```python
from build123d import *

# Parameters (mm, degrees)
SKETCH_R           = 64
PAD_DEPTH          = 4
PAD001_DEPTH       = 50
POLARPATTERN_COUNT = 3
SKETCH002_R        = 64
PAD002_DEPTH       = 4


with BuildPart() as part:
    # Sketch → Pad (new body)
    with BuildSketch(Plane.XY):
        Circle(SKETCH_R)
    extrude(amount=-PAD_DEPTH)

    # Sketch001 → Pad001 (join)
    with BuildSketch(Plane.XY):
        with BuildLine():
            ThreePointArc((29, 19.052559), (29, -19.052559), (62, 0))
            ThreePointArc((62, 0), (60, 2), (58, 0))
            ThreePointArc((31, 15.588457), (31, -15.588457), (58, 0))
            ThreePointArc((31, 15.588457), (41.999973, 34.641035), (30.99994, 53.693578))
            ThreePointArc((30.99994, 53.693578), (28.267891, 52.961523), (28.999946, 50.229473))
            ThreePointArc((29, 19.052559), (37.999973, 34.641032), (28.999946, 50.229473))
        make_face()
    pad001 = extrude(amount=PAD001_DEPTH)

    # PolarPattern: Pad001 ×3 about axis
    polarpattern_axis = Axis((0, 0, 0), (0, 0, 1))
    for i in range(1, POLARPATTERN_COUNT):
        add(pad001.rotate(polarpattern_axis, i * 360 / POLARPATTERN_COUNT))

    # Sketch002 → Pad002 (join)
    with BuildSketch(Plane.XY.offset(50)):
        Circle(SKETCH002_R)
    extrude(amount=PAD002_DEPTH)


solid = part.part
```
The model under review builds one solid part; all positions refer to its coordinate system, in mm. A direction names the side the tool comes from. Round coordinates to 2 decimals unless told otherwise and drop trailing zeros. Order: outer loops, then holes, each group sorted by start corner. A loop starts at its lowest first (then second) coordinate and runs counter-clockwise, first axis right, second up.
(1) Take a section at D-D, the plane x = -12.5. State the section outline as (y, z) points, plus the area to 3 significant figures.
Working result:
outline: (-62.77, -4) - (62.77, -4) - (62.77, 0) - (55.32, 0) - (55.32, 50) - (62.77, 50) - (62.77, 54) - (-62.77, 54) - (-62.77, 50) - (-18.28, 50) - (-18.28, 0) - (-62.77, 0) - close; hole (-13.96, 0) - (13.96, 0) - (13.96, 50) - (-13.96, 50) - close; hole (18.28, 0) - (51, 0) - (51, 50) - (18.28, 50) - close
area: 1,650 mm2
(2) Take a section at A-A, the plane z = 46. State the section outline as (x, y) points.
Working result:
outline: (-62, 0) arc R2 ccw to (-58, 0) arc R18 cw to (-31, 15.59) arc R22 ccw (long way) to (-31, 53.69) arc R2 ccw to (-29, 50.23) arc R18 cw (long way) to (-29, 19.05) arc R22 ccw to start; (-31, -53.69) arc R2 ccw to (-29, -50.23) arc R18 cw (long way) to (-2, -34.64) arc R22 ccw to (31, -53.69) arc R2 ccw to (29, -50.23) arc R18 cw to (2, -34.64) arc R22 ccw (long way) to start; (29, 19.05) arc R22 ccw (long way) to (62, 0) arc R2 ccw to (58, 0) arc R18 cw (long way) to (31, 15.59) arc R22 ccw to (31, 53.69) arc R2 ccw to (29, 50.23) arc R18 cw to start
(3) For P1, Ø1, axis at x = -14, z = 21.5, coming from the -Y side; P2, Ø1.5, axis at y = 49.5, z = 28, coming from the +X side, all flat-tipped, find the tip position at first contact; note any pin that passes through.
Working result:
P1: stops at y = -17.86
P2: stops at x = 36.88
(4) Take a section at C-C, the plane y = 24. State the section outline as (x, z) points.
Working result:
outline: (-59.33, -4) - (59.33, -4) - (59.33, 0) - (39.26, 0) - (39.26, 50) - (59.33, 50) - (59.33, 54) - (-59.33, 54) - (-59.33, 50) - (-5.48, 50) - (-5.48, 0) - (-59.33, 0) - close; hole (-0.74, 0) - (34.52, 0) - (34.52, 50) - (-0.74, 50) - close
(5) Wall thickness on L1, parallel to Y at x = -20, z = 18; L2, parallel to Z at x = -47, y = 3; L3, parallel to X at y = -0.5, z = 22: over which ranges is each line inside the solid? List them lowest first.
Working result:
L1: y = -16.64 to -12.64, 12.64 to 16.64, 52.64 to 56.64
L2: z = -4 to 0, 50 to 54
L3: x = -61.94 to -58.06, 18.01 to 22.01, 57.99 to 61.99
(6) Mouldability with a two-part tool opening along Y and no side actions: class faces 1 (the face through (-60, -2, 25)), 2 (the face through (-13.87, -62.48, -1.97)), 3 (the face through (-1, 1, 50)), 4 (the face through (1.99, 34, 24.65)) as released by +Y, released by -Y, zero draft, split by the parting line, or undercut.
Working result:
face 1: released by -Y
face 2: split by the parting line
face 3: undercut
face 4: undercut
(7) Tool access review of faces 5 (the face through (41.998, 34.319, 24.65)), 6 (the face through (-2.008, 34.113, 24.65)), 7 (the face through (60, 2, 25)): name each direction out of +Z, -Z, +X, -X, +Y, -Y from which nothing blocks a thin tool from reaching the whole face with its end or side.
Working result:
face 5: +X
face 6: none
face 7: +Y
(8) Take a section at B-B, the plane x = -40. State the section outline as (y, z) points, plus the area to 3 significant figures.
Working result:
outline: (-49.96, -4) - (49.96, -4) - (49.96, 0) - (22, 0) - (22, 50) - (49.96, 50) - (49.96, 54) - (-49.96, 54) - (-49.96, 50) - (-43.81, 50) - (-43.81, 0) - (-49.96, 0) - close; hole (-25.48, 0) - (18, 0) - (18, 50) - (-25.48, 50) - close
area: 1,920 mm2
